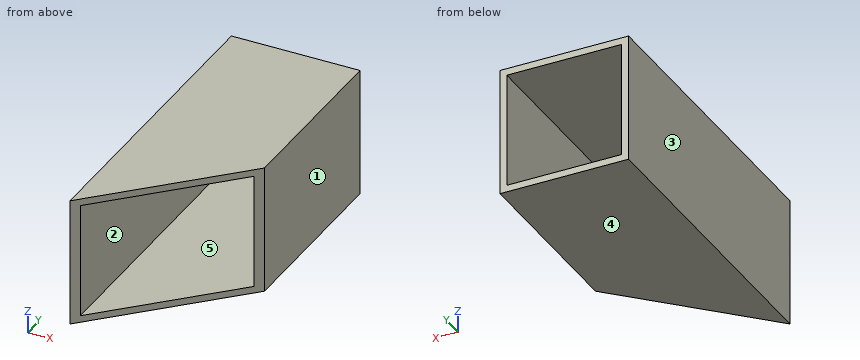
from build123d import *

# Parameters (mm, degrees)
CROQUIS1_W              = 56.5
CROQUIS1_H              = 56.5
SALIENTE_EXTRUIR1_DEPTH = 81.9
SALIENTE_EXTRUIR2_DEPTH = 56.5
VACIADO4_T              = -3


with BuildPart() as part:
    # Croquis1 → Saliente-Extruir1 (new body)
    with BuildSketch(Plane(origin=(0, 0, 0), x_dir=(1, 0, 0), z_dir=(0, 1, 0))):
        with Locations((28.25, 28.25)):
            Rectangle(CROQUIS1_W, CROQUIS1_H)
    extrude(amount=SALIENTE_EXTRUIR1_DEPTH)

    # Croquis2 → Saliente-Extruir2 (add)
    with BuildSketch(Plane.XY):
        Polygon((0, 0), (0, -56.5), (56.5, 0), align=None)
    extrude(amount=-SALIENTE_EXTRUIR2_DEPTH)

    # Vaciado4
    vaciado4_openings = [part.faces().sort_by_distance(p)[0] for p in [
        (28.25, 81.9, -28.25),
        (28.25, -28.25, -28.25),
    ]]
    offset(amount=VACIADO4_T, openings=vaciado4_openings, kind=Kind.INTERSECTION)


solid = part.part
For this review, take the finished solid that the model builds, in its own axes (mm). Face numbers are marked on the shaded views. A direction names the side the tool comes from. Coordinates: 2 decimals unless noted, no trailing zeros. Loops run counter-clockwise (first coordinate to the right, second up) from the corner with the lowest first, then second, coordinate; pieces in that order, holes last. Notation, with made-up numbers: (19.25, -36) - (62.25, -36) arc R33 ccw to (62.25, 3) - close; hole circle Ø9 at (-21.75, 85). An arc over 180 degrees is marked (long way). Use a Markdown table: item, result. Add a question column.
Item 1: For line 1 (X direction, y = 52, z = -50.5); line 2 (Z direction, x = 35.5, y = -20); line 3 (X direction, y = -24.5, z = -19), list the stretches that pass through material, from the lowest coordinate up.
Item 2: Mouldability with a two-part tool opening along X and no side actions: class the marked faces 3, 4 and 5 as pulls with the +X half, pulls with the -X half, needs draft (parallel to the pull), parting line crosses it, or undercut.
Item 3: We need section A-A (x = 48.5). Give the boundary of the cut face in (y, z).
Item 4: We need section C-C (z = -28). Give the boundary of the cut face in (x, y).
Item 5: Tool access review of the marked faces 1 and 2: name each direction out of +Z, -Z, +X, -X, +Y, -Y from which nothing blocks a thin tool from reaching the whole face with its end or side.
Item 6: We need section B-B (y = -41). Give the boundary of the cut face in (x, z).
Item 7: We need section D-D (y = 21.5). Give the boundary of the cut face in (x, z), and give its area (3 significant figures).
Results list:
| question | item | result |
|---|---|---|
| 1 | line 1 | x = 0 to 3, 53.5 to 56.5 |
| 1 | line 2 | z = -56.5 to -53.5, -3 to 0 |
| 1 | line 3 | x = 0 to 3 |
| 2 | face 3 | pulls with the -X half |
| 2 | face 4 | needs draft |
| 2 | face 5 | undercut |
| 3 | outline | (-8, -56.5) - (81.9, -56.5) - (81.9, -53.5) - (-8, -53.5) - close; (-8, -3) - (81.9, -3) - (81.9, 0) - (-8, 0) - close |
| 4 | outline | (0, -56.5) - (3, -53.5) - (3, 81.9) - (0, 81.9) - close; (53.5, -3) - (56.5, 0) - (56.5, 81.9) - (53.5, 81.9) - close |
| 5 | face 1 | +Z, -Z, +X, +Y, -Y |
| 5 | face 2 | +Y, -Y |
| 6 | outline | (0, -56.5) - (15.5, -56.5) - (15.5, -53.5) - (3, -53.5) - (3, -3) - (15.5, -3) - (15.5, 0) - (0, 0) - close |
| 7 | outline | (0, -56.5) - (56.5, -56.5) - (56.5, 0) - (0, 0) - close; hole (3, -53.5) - (53.5, -53.5) - (53.5, -3) - (3, -3) - close |
| 7 | area | 642 mm^2 |
